Autodesk Inventor part; units mm, degrees
ref_plane "YZ Plane" through (0, 0, 0) normal (1, 0, 0) x (0, 1, 0)
ref_plane "XZ Plane" through (0, 0, 0) normal (0, 1, 0) x (-1, 0, 0)
ref_plane "XY Plane" through (0, 0, 0) normal (0, 0, 1) x (1, 0, 0)
sketch "Sketch1" plane through (0, 0, 0) normal (1, 0, 0) x (0, 1, 0)
  line L0 (20, 18) -> (-20, 18)
  line L1 (-20, 18) -> (-20, -18)
  line L2 (-20, -18) -> (20, -18)
  line L3 (20, -18) -> (20, 18)
  line L4 (13, -10) -> (-13, -10)
  line L5 (-13, -10) -> (-13, 10)
  line L6 (-13, 10) -> (13, 10)
  line L7 (13, 10) -> (13, -10)
  line L8 (20, 0) -> (-20, 0) construction
  line L9 (0, -18) -> (0, 18) construction
  circle A0 centre (16, 6) radius 1.5
  circle A1 centre (16, -6) radius 1.5
  circle A2 centre (-16, 6) radius 1.5
  circle A3 centre (-16, -6) radius 1.5
  circle A4 centre (8, 13) radius 1.5
  circle A5 centre (8, -13) radius 1.5
  circle A6 centre (-8, 13) radius 1.5
  circle A7 centre (-8, -13) radius 1.5
  point P0 (0, 0)
  dimension "d0" = 40
  dimension "d1" = 36
  dimension "d2" = 26
  dimension "d3" = 20
  dimension "d5" = 3
  dimension "d6" = 6
  dimension "d7" = 16
  dimension "d8" = 3
  dimension "d9" = 8
  dimension "d10" = 13
  dimension "d17" = 7
  dimension "d18" = 8
  dimension "d19" = 20
  dimension "d20" = 18
extrude "Extrusion1" add sketch "Sketch1" along normal blind 16
sketch "Sketch2" plane through (0, -20, -18) normal (0, -1, 0) x (1, 0, 0)
  line L0 (0, 36) -> (16, 36) construction
  line L1 (8, 36) -> (8, 0) construction
  line L2 (0, 0) -> (16, 0) construction
  line L3 (16, 8) -> (16, 28) construction
  line L4 (16, 18) -> (0, 18) construction
  line L5 (8, 18) -> (8, 28) construction
  line L6 (8, 28) -> (8, 8) construction
  line L7 (8, 18) -> (14, 18) construction
  line L8 (14, 18) -> (2, 18) construction
  ellipse E0 centre (8, 18) end of major axis (14, 18) minor radius 10 construction
  ellipse E1 centre (8, 18) end of major axis (14, 18) minor radius 10
  dimension "d13" = 10
  dimension "d14" = 20
  dimension "d15" = 6
  dimension "d16" = 12
extrude "Extrusion2" add sketch "Sketch2" along normal blind 8
sketch "Sketch3" plane through (0, -28, -18) normal (0, -1, 0) x (1, 0, 0)
  ellipse E0 centre (8, 18) end of major axis (8, 28) minor radius 6 construction
  line L0 (8, 28) -> (8, 8) construction
  circle A0 centre (8, 25) radius 1.25
  circle A1 centre (8, 11) radius 1.25
  point P0 (0, 18)
  dimension "d23" = 2.5
  dimension "d24" = 7
  dimension "d25" = 2.5
  dimension "d26" = 7
  dimension "d27" = 0
extrude "Extrusion3" cut sketch "Sketch3" against normal blind 6
thread "Thread1"
thread "Thread2"
sketch "Sketch4" plane through (0, -28, -18) normal (0, -1, 0) x (1, 0, 0)
  ellipse E0 centre (8, 18) end of major axis (8, 28) minor radius 6 construction
  line L0 (14, 18) -> (8, 18) construction
  circle A0 centre (8, 18) radius 2.5
  point P0 (0, 18)
  dimension "d34" = 5
extrude "Extrusion4" cut sketch "Sketch4" against normal blind 90
sketch "Sketch5" plane through (0, -28, -18) normal (0, -1, 0) x (1, 0, 0)
  circle A0 centre (8, 18) radius 2.5 construction
  line L0 (5.5, 18) -> (8, 18) construction
  circle A1 centre (8, 18) radius 4
  point P0 (0, 18)
  dimension "d37" = 8
extrude "Extrusion5" cut sketch "Sketch5" against normal blind 8
chamfer "Chamfer1" distance 1 angle 45 2 edges at (6.75, -22, 7) (6.75, -22, -7)
chamfer "Chamfer2" distance 1 angle 45 1 edges at (4, -20, 0)
sketch "Sketch6" plane through (0, -20, 18) normal (0, 0, 1) x (1, 0, 0)
  line L0 (0, 40) -> (16, 40) construction
  line L1 (8, 40) -> (8, 0) construction
  line L2 (0, 0) -> (16, 0) construction
  circle A0 centre (8, 20) radius 2.5 construction
  circle A1 centre (8, 20) radius 2.5
  point P0 (0, 20)
  dimension "d46" = 5
extrude "Extrusion6" cut sketch "Sketch6" against normal blind 6
sketch "Sketch7" plane through (8, 0, 12) normal (0, 0, 1) x (1, 0, 0)
  circle A0 centre (0, 0) radius 1.5
  line L0 (-8, -13) -> (8, -13)
  point P0 (-8, 0)
  dimension "d49" = 3
  dimension "d50" = 8
  dimension "d51" = 13
extrude "Extrusion7" cut sketch "Sketch7" against normal blind 6
chamfer "Chamfer3" distance 1 angle 45 1 edges at (6.5, 0, 12)
thread "Thread3"
sketch "Sketch8" plane through (0, 20, 18) normal (0, 1, 0) x (1, 0, 0)
  circle A0 centre (8, 18) radius 2.5 construction
  line L0 (5.5, 18) -> (8, 18) construction
  circle A1 centre (8, 18) radius 4
  point P0 (0, 18)
  dimension "d59" = 8
extrude "Extrusion8" add sketch "Sketch8" along normal blind 10
fillet "Fillet1" radius 4 1 edges at (4, 30, 0)
fillet "Fillet2" radius 2 1 edges at (4, 20, 0)
sketch "Sketch9" plane through (0, 13, -10) normal (0, -1, 0) x (1, 0, 0)
  circle A0 centre (8, 10) radius 2.5 construction
  line L0 (5.5, 10) -> (8, 10) construction
  circle A1 centre (8, 10) radius 2.5
  point P0 (0, 10)
extrude "Extrusion9" cut sketch "Sketch9" against normal blind 16
fillet "Fillet3" radius 2 1 edges at (5.5, 29, 0)
properties part number "Steam Chest" material "Iron, Cast"
Read the model definition and answer for the solid it produces. Units are mm, in the model's axes. A direction names the side the tool comes from. Coordinates: 2 decimals unless noted, no trailing zeros. Order: outer loops, then holes, each group sorted by start corner. A loop starts at its lowest first (then second) coordinate and runs counter-clockwise, first axis right, second up. Notation, with made-up numbers: M 24.5,86.5 L 76.5,86.5 A30 cw 76.5,113.5 Z; hole C 17.25,84.5 d4. An arc over 180 degrees is marked long. Put each result on its own line as item: value. Start each with the question number.
Item 1: Section D-D, the plane z = 13 is taken. Determine the outline of the cut face in (x, y), plus the area to 3 significant figures.
Item 2: Section B-B, the plane z = -13 is taken. Determine the outline of the cut face in (x, y).
Item 3: Section A-A, the plane y = -16 is taken. Determine the outline of the cut face in (x, z), plus the area to 3 significant figures.
Item 4: The mould has two halves that part along X. Classify faces 1 (the face through (16, 0, -12)), 2 (the face through (7.9, -28, -4.3)), 3 (the face through (10.385, 0.751, 15.042)): +X half, -X half, draft (parallel to the pull), parting line (faces both ways), or undercut.
Item 5: Given pin 1 Ø1.8 at (y, z) = (16, 6) entering from +X; pin 2 Ø5 at (x, z) = (5.5, -4.5) entering from +Y; pin 3 Ø1.5 at (x, z) = (8, 7) entering from -Y; pin 4 Ø0.5 at (x, z) = (8, 0) entering from -Y, each flat-ended and moving along its own axis, determine where each tip first touches the part or whether it passes through.
Item 6: Consider probe 1 along Z at (x, y) = (7, 8); probe 2 along Z at (x, y) = (8, -25.25); probe 3 along Z at (x, y) = (11, 16). Determine where each line is inside the solid, lowest interval first. Write a range as [from, to].
Item 7: For faces 4 (the face through (4, 0, 18)), 5 (the face through (6.5, 0.07, 10.51)), 6 (the face through (4.8, -24.5, -2.4)), 7 (the face through (6, 0, 10)), 8 (the face through (8, 0, -18)), determine the directions among +Z, -Z, +X, -X, +Y, -Y from which every point of the face is accessible in a straight line to the end or side of a thin tool.
Item 8: Section C-C, the plane y = 0 is taken. Count the separate pieces of the cut face and the enclosed holes in it, plus the area to 3 significant figures.
Computed:
1. outline: M 0,-20 L 16,-20 L 16,-9.5 L 0,-9.5 Z; M 0,-6.5 L 16,-6.5 L 16,6.5 L 0,6.5 Z; M 0,9.5 L 16,9.5 L 16,20 L 0,20 Z; hole C 8,0 d5
1. area: 524 mm2
2. outline: M 0,-20 L 16,-20 L 16,-9.5 L 0,-9.5 Z; M 0,-6.5 L 16,-6.5 L 16,6.5 L 0,6.5 Z; M 0,9.5 L 16,9.5 L 16,20 L 0,20 Z
3. outline: M 0,-18 L 16,-18 L 16,-7.5 L 0,-7.5 Z; M 0,-4.5 L 16,-4.5 L 16,4.5 L 0,4.5 Z; M 0,7.5 L 16,7.5 L 16,18 L 0,18 Z; hole C 8,0 d5
3. area: 460 mm2
4. face 1: +X half
4. face 2: draft
4. face 3: undercut
5. pin 1: passes through
5. pin 2: stops at y = 29
5. pin 3: stops at y = -22.5
5. pin 4: stops at y = 29
6. probe 1: z = [-18, -14.5], [-11.5, -10], [10, 11.5], [14.5, 18]
6. probe 2: z = [-10, -8.25], [-5.75, -4], [4, 5.75], [8.25, 10]
6. probe 3: z = [-18, -7.5], [-4.5, 4.5], [7.5, 18]
7. face 4: +Z, +X, -X, +Y, -Y
7. face 5: +Z
7. face 6: -Y
7. face 7: +X, -X
7. face 8: -Z, +X, -X, +Y, -Y
8. separate pieces: 3
8. enclosed holes: 0
8. area: 219 mm2
